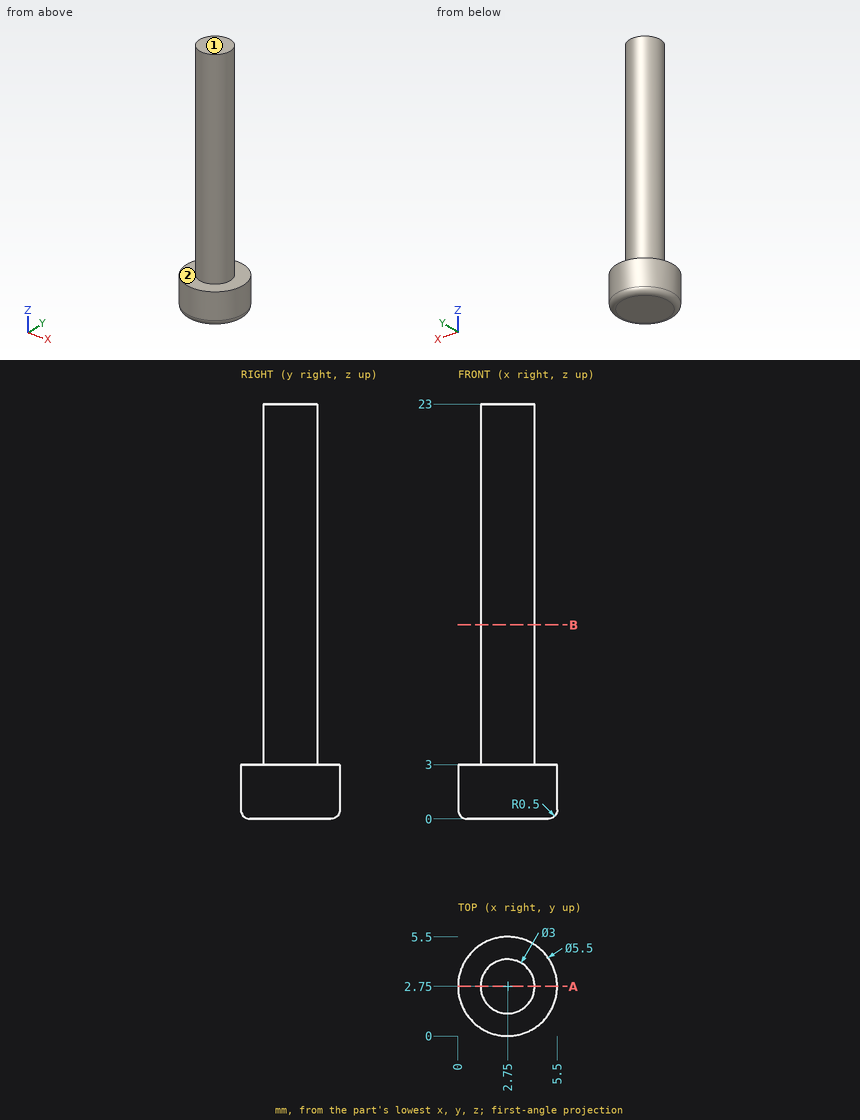
Answer from the drawing. Dimensions are ordinates in mm from the lowest x, y and z of the part. A direction names the side the tool comes from. Coordinates: 2 decimals unless noted, no trailing zeros. Order: outer loops, then holes, each group sorted by start corner. A loop starts at its lowest first (then second) coordinate and runs counter-clockwise, first axis right, second up. Notation, with made-up numbers: (41.5, 54) - (52.5, 54) arc R25 ccw to (52.5, 76) - close; hole circle Ø10 at (12, 33). An arc over 180 degrees is marked (long way). Put each result on its own line as item: value. Start each with the question number.
1) Find section A-A (y = 2.75). Give the vertices of the cut face in (x, z), plus the area to 3 significant figures.
2) Find section B-B (z = 10.75). Give the vertices of the cut face in (x, y).
3) Find the intervals of material crossed by line 1 (Z direction, x = 5, y = 2.3); line 2 (Y direction, x = 2.1, z = 21); line 3 (X direction, y = 3.9, z = 7.75), in increasing order. Write a range as from..to.
4) For the marked faces 1 and 2, determine the directions among +Z, -Z, +X, -X, +Y, -Y from which every point of the face is accessible in a straight line to the end or side of a thin tool.
5) Flat-ended cylindrical pins translate along their axes: pin 1 (3 mm diameter, centred on x = 1.5, y = 4, fed in from -Z); pin 2 (3 mm diameter, centred on y = 4.5, z = 16, fed in from +X); pin 3 (1 mm diameter, centred on x = 4.5, y = 0.5, fed in from +Z); pin 4 (3 mm diameter, centred on x = 3.5, z = 15, fed in from -Y). Find the tip coordinate at first contact, or state that the pin passes through.
Results list:
1. outline: (0, 0.5) arc R0.5 ccw to (0.5, 0) - (5, 0) arc R0.5 ccw to (5.5, 0.5) - (5.5, 3) - (4.25, 3) - (4.25, 23) - (1.25, 23) - (1.25, 3) - (0, 3) - close
1. area: 76.4 mm^2
2. outline: circle Ø3 at (2.75, 2.75)
3. line 1: z = 0..3
3. line 2: y = 1.4..4.1
3. line 3: x = 1.79..3.71
4. face 1: +Z, +X, -X, +Y, -Y
4. face 2: +Z
5. pin 1: stops at z = 0
5. pin 2: stops at x = 4.23
5. pin 3: stops at z = 3
5. pin 4: stops at y = 1.25
